Model file for the job. Use its own axes, mm. A direction names the side the tool comes from. Round coordinates to 2 decimals unless told otherwise and drop trailing zeros. Loops run counter-clockwise (first coordinate to the right, second up) from the corner with the lowest first, then second, coordinate; pieces in that order, holes last.
from build123d import *
from build123d.topology import SkipClean

# Parameters (mm, degrees)
SZKIC1_R                         = 10
DODANIE_WYCI_GNI_CIE1_DEPTH      = 60
SZKIC3_R                         = 6
WYTNIJ_WYCI_GNI_CIE1_DEPTH       = 50
WYTNIJ_WYCI_GNI_CIE2_DEPTH       = 20
SZKIC9_R                         = 32.5
SZKIC9_R_2                       = 3
SZKIC9_R_3                       = 10
DODANIE_WYCI_GNI_CIE3_DEPTH      = 10
SZKIC12_R                        = 10
DODANIE_WYCI_GNI_CIE4_DEPTH      = 10
DODANIE_WYCI_GNI_CIE6_DEPTH      = 4
DODANIE_WYCI_GNI_CIE6_DEPTH_BACK = 10
SZKIC13_R                        = 16
SZKIC13_R_2                      = 10
SZKIC14_W                        = 1.3
SZKIC14_H                        = 0.5
FILLET3_R                        = 4
WYTNIJ_WYCI_GNI_CIE4_START       = -5
WYTNIJ_WYCI_GNI_CIE4_DEPTH       = 15
CUT_EXTRUDE1_DEPTH               = 84.740671122
CUT_EXTRUDE1_DEPTH_BACK          = 84.740671122
FILLET1_R                        = 0.8
CIRPATTERN1_COUNT                = 4
PRZENIE_CIAN_1_OUTLINE_W         = 0.5
PRZENIE_CIAN_1_OUTLINE_H         = 1.3
PRZENIE_CIAN_1_2_OUTLINE_W       = 0.5
PRZENIE_CIAN_1_2_OUTLINE_H       = 1.3
PRZENIE_CIAN_2_BY                = 3


with BuildPart() as part:
    # Szkic1 → Dodanie-wyciągnięcie1 (new body)
    with BuildSketch(Plane.XY):
        Circle(SZKIC1_R)
    extrude(amount=DODANIE_WYCI_GNI_CIE1_DEPTH)

    # Szkic3 → Wytnij-wyciągnięcie1 (cut)
    with BuildSketch(Plane.XY.offset(60)):
        Circle(SZKIC3_R)
    extrude(amount=-WYTNIJ_WYCI_GNI_CIE1_DEPTH, mode=Mode.SUBTRACT)

    # Szkic8 → Wytnij-wyciągnięcie2 (cut)
    with BuildSketch(Plane.XY.offset(60)):
        with BuildLine():
            Line((0, 8), (0, 6))
            ThreePointArc((0, 6), (1.014611872, 5.913591358), (2, 5.656854249))
            Line((2, 5.656854249), (2, 8))
            Line((2, 8), (0, 8))
        make_face()
        with BuildLine():
            ThreePointArc((-2, 5.656854249), (-1.014611872, 5.913591358), (0, 6))
            Line((0, 6), (0, 8))
            Line((0, 8), (-2, 8))
            Line((-2, 8), (-2, 5.656854249))
        make_face()
    extrude(amount=-WYTNIJ_WYCI_GNI_CIE2_DEPTH, mode=Mode.SUBTRACT)


with BuildPart() as body_2:
    # Szkic9 → Dodanie-wyciągnięcie3 (new body)
    with BuildSketch(Plane(origin=(0, 0, 0), x_dir=(-1, 0, 0), z_dir=(0, 0, -1))):
        Circle(SZKIC9_R)
        with Locations((0, 25)):
            Circle(SZKIC9_R_2, mode=Mode.SUBTRACT)
        with Locations((-25, 0)):
            Circle(SZKIC9_R_2, mode=Mode.SUBTRACT)
        with Locations((0, -25)):
            Circle(SZKIC9_R_2, mode=Mode.SUBTRACT)
        with Locations((25, 0)):
            Circle(SZKIC9_R_2, mode=Mode.SUBTRACT)
        with Locations(Location((0, 0, 0), (0, 0, 180))):
            Circle(SZKIC9_R_3, mode=Mode.SUBTRACT)
    extrude(amount=DODANIE_WYCI_GNI_CIE3_DEPTH)


with BuildPart() as dodanie_wyci_gni_cie4_tool:
    # Szkic12 → Dodanie-wyciągnięcie4 (new body)
    with BuildSketch(Plane(origin=(0, 0, -10), x_dir=(-1, 0, 0), z_dir=(0, 0, -1))):
        Circle(SZKIC12_R)
    extrude(amount=-DODANIE_WYCI_GNI_CIE4_DEPTH)


with BuildPart() as part_1:
    add(part.part)


with BuildPart() as part_2:
    # Dodanie-wyciągnięcie4: joined with dodanie_wyci_gni_cie4_tool
    add(part_1.part.fuse(dodanie_wyci_gni_cie4_tool.part, body_2.part, tol=0.00001))

    # Szkic13 → Dodanie-wyciągnięcie6 (add, two sides: drawn at the far end of the back side and taken through both)
    with BuildSketch(Plane.XY.offset(10).offset(-DODANIE_WYCI_GNI_CIE6_DEPTH_BACK)):
        Circle(SZKIC13_R)
        Circle(SZKIC13_R_2, mode=Mode.SUBTRACT)
    extrude(amount=DODANIE_WYCI_GNI_CIE6_DEPTH + DODANIE_WYCI_GNI_CIE6_DEPTH_BACK)

    # Szkic14 → Wycięcie-obrót1 (revolve, cut)
    with BuildSketch(Plane(origin=(0, 0, 0), x_dir=(0, 0, -1), z_dir=(1, 0, 0)), mode=Mode.PRIVATE) as wyci_cie_obr_t1_sk:
        with Locations((-32.65, 9.75)):
            Rectangle(SZKIC14_W, SZKIC14_H)
    revolve(wyci_cie_obr_t1_sk.sketch.rotate(Axis((0, 0, 10), (0, 0, 1)), 90), axis=Axis((0, 0, 10), (0, 0, 1)), mode=Mode.SUBTRACT)

    # Fillet3
    fillet3_edges = [part_2.edges().sort_by_distance(p)[0] for p in [
        (-16, 0, 0),
    ]]
    fillet(fillet3_edges, radius=FILLET3_R)

    # Szkic15 → Wytnij-wyciągnięcie4 (cut)
    with SkipClean():  # the faces are left unmerged after this step: merging them gives an invalid solid
        with BuildSketch(Plane.XY.offset(WYTNIJ_WYCI_GNI_CIE4_START)):
            with BuildLine():
                Line((-21, 5), (-38.344899327, 5))
                Line((-38.344899327, 5), (-38.344899327, -5))
                Line((-38.344899327, -5), (-21, -5))
                ThreePointArc((-21, -5), (-16, 0), (-21, 5))
            make_face()
        wytnij_wyci_gni_cie4 = extrude(amount=WYTNIJ_WYCI_GNI_CIE4_DEPTH, mode=Mode.SUBTRACT)

    # Sketch1 → Cut-Extrude1 (cut, two sides: drawn at the far end of the back side and taken through both)
    with SkipClean():  # the faces are left unmerged after this step: merging them gives an invalid solid
        with BuildSketch(Plane.XY.offset(60).offset(-CUT_EXTRUDE1_DEPTH_BACK)):
            with BuildLine():
                ThreePointArc((2, 5.656854249), (0, 6), (-2, 5.656854249))
                ThreePointArc((-2, 5.656854249), (-3.464101615, -4.898979486), (6, 0))
                ThreePointArc((6, 0), (4.898979486, 3.464101615), (2, 5.656854249))
            make_face()
            with BuildLine():
                Line((2, 8), (-2, 8))
                Line((-2, 8), (-2, 5.656854249))
                ThreePointArc((-2, 5.656854249), (0, 6), (2, 5.656854249))
                Line((2, 5.656854249), (2, 8))
            make_face()
        extrude(amount=CUT_EXTRUDE1_DEPTH + CUT_EXTRUDE1_DEPTH_BACK, mode=Mode.SUBTRACT)

    # Fillet1
    fillet1_edges = [part_2.edges().sort_by_distance(p)[0] for p in [
        (-10, 0, 14),
    ]]
    fillet(fillet1_edges, radius=FILLET1_R)

    # CirPattern1: Wytnij-wyciągnięcie4 ×4 about axis
    cirpattern1_axis = Axis((0, 0, 0), (0, 0, 1))
    for i in range(1, CIRPATTERN1_COUNT):
        add(wytnij_wyci_gni_cie4.rotate(cirpattern1_axis, i * 360 / CIRPATTERN1_COUNT), mode=Mode.SUBTRACT)

    # Przenieś ścianę1: read off the stored shape, not the designer's step
    # Przenieś ścianę1 outline → Przenieś ścianę1 (revolve, cut)
    with BuildSketch(Plane.XZ):
        with Locations((9.75, 41.65)):
            Rectangle(PRZENIE_CIAN_1_OUTLINE_W, PRZENIE_CIAN_1_OUTLINE_H)
    revolve(axis=Axis((0, 0, 0), (0, 0, 1)), mode=Mode.SUBTRACT)

    # Przenie_ _cian_1 2 outline → Przenie_ _cian_1 2 (revolve)
    with BuildSketch(Plane.XZ):
        with Locations((9.75, 32.65)):
            Rectangle(PRZENIE_CIAN_1_2_OUTLINE_W, PRZENIE_CIAN_1_2_OUTLINE_H)
        with BuildLine():
            ThreePointArc((10.8, 23), (10.234314575, 23.234314575), (10, 23.8))
            Line((10, 23.8), (10, 14.8))
            ThreePointArc((10, 14.8), (10.234314575, 14.234314575), (10.8, 14))
            Line((10.8, 14), (16, 14))
            Line((16, 14), (16, 23))
            Line((16, 23), (10.8, 23))
        make_face()
    revolve(axis=Axis((0, 0, 0), (0, 0, 1)))

    # Przenieś ścianę2: a face moved outward by 3.0
    extrude(part_2.faces().sort_by_distance((0, -8, 60))[0], amount=PRZENIE_CIAN_2_BY, dir=(0, 0, 1))


solid = part_2.part
Q1. Slice it at D-D on z = 40. Give the cut face in (x, y), plus the area to 3 significant figures.
Q2. Tool access for faces 1 (the face through (19, 19, 0)), 2 (the face through (22.5, -2.3, -5)), 3 (the face through (5, -27, -3)), 4 (the face through (-27, -5, -3)): list every direction of +Z, -Z, +X, -X, +Y, -Y with a clear straight run to the whole face (end or side of a thin tool).
Q3. Pull direction X, two halves, no side cores. Call faces 5 (the face through (-16, 0, -2)), 6 (the face through (-2.3, -22.5, -5)), 7 (the face through (-2.17, -9.76, 52.51)), 8 (the face through (0, -7, -10)): pulls with the +X half, pulls with the -X half, needs draft (parallel to the pull), parting line crosses it, or undercut.
Q4. Slice it at C-C on z = -3. Give the cut face in (x, y).
Q5. Slice it at A-A on y = -25. Give the cut face in (x, z), plus the area to 3 significant figures.
Q6. Probe line 1 (Y direction, x = 0, z = -6.75); line 2 (Y direction, x = 0, z = 50); line 3 (Z direction, x = -9.5, y = 10.5). List the from-to ranges inside material, lowest first.
Q7. Flat gauge pins, fed straight in: P1, Ø4, axis at x = -29, z = -3, coming from the +Y side; P2, Ø13.5, axis at x = -23, y = -17.5, coming from the +Z side; P3, Ø4, axis at y = 28, z = -1.5, coming from the +X side; P4, Ø5.5, axis at x = 0, y = -25, coming from the +Z side. Where does each tip first touch, or does it go through?
Q8. Slice it at B-B on x = 24. Give the cut face in (y, z).
Reply:
1. outline: circle Ø20 at (0, 0); hole (-2, 5.66) arc R6 ccw (long way) to (2, 5.66) - (2, 8) - (-2, 8) - close
1. area: 193 mm2
2. face 1: +Z, +X, +Y
2. face 2: +Z, +X
2. face 3: +Z, -Y
2. face 4: +Z, -X
3. face 5: pulls with the -X half
3. face 6: undercut
3. face 7: parting line crosses it
3. face 8: needs draft
4. outline: (-32.11, -5) arc R32.5 ccw to (-5, -32.11) - (-5, -21) arc R5 cw to (5, -21) - (5, -32.11) arc R32.5 ccw to (32.11, -5) - (21, -5) arc R5 cw to (21, 5) - (32.11, 5) arc R32.5 ccw to (5, 32.11) - (5, 21) arc R5 cw to (-5, 21) - (-5, 32.11) arc R32.5 ccw to (-32.11, 5) - (-21, 5) arc R5 cw to (-21, -5) - close; hole (-2, 5.66) arc R6 ccw (long way) to (2, 5.66) - (2, 8) - (-2, 8) - close
5. outline: (-20.77, -10) - (-3, -10) - (-3, -5) - (-5, -5) - (-5, 0) - (-20.77, 0) - close; (3, -10) - (20.77, -10) - (20.77, 0) - (5, 0) - (5, -5) - (3, -5) - close
5. area: 335 mm2
6. line 1: y = -32.5 to -28, -22 to -6, 8 to 22, 28 to 32.5
6. line 2: y = -10 to -6, 8 to 10
6. line 3: z = -10 to 23
7. P1: stops at y = 18.09
7. P2: stops at z = 0
7. P3: stops at x = 19.5
7. P4: passes through
8. outline: (-21.91, -10) - (-2.83, -10) - (-2.83, -5) - (-5, -5) - (-5, 0) - (-21.91, 0) - close; (2.83, -10) - (21.91, -10) - (21.91, 0) - (5, 0) - (5, -5) - (2.83, -5) - close
